```python
from build123d import *

# Parameters (mm, degrees)
SKETCH1_R           = 1.5
BOSS_EXTRUDE1_DEPTH = 5.13
SKETCH2_W           = 21.373732632
SKETCH2_H           = 5.13
BOSS_EXTRUDE2_DEPTH = 2.5
SKETCH3_W           = 21.373732632
SKETCH3_H           = 2.5
BOSS_EXTRUDE3_DEPTH = 4.6
BOSS_EXTRUDE4_START = -2.95
BOSS_EXTRUDE4_DEPTH = 2.95
CUT_EXTRUDE1_REACH  = 103.599
SKETCH5_R           = 1.75
SKETCH6_R           = 1.6
SKETCH6_R_2         = 1.5
CUT_EXTRUDE2_DEPTH  = 34.549423701
CUT_EXTRUDE3_REACH  = 103.262


with BuildPart() as part:
    # Sketch1 → Boss-Extrude1 (new body)
    with BuildSketch(Plane.XY):
        with BuildLine():
            Line((-11.282357346, 86.580844321), (-10.686866316, 72.941857381))
            Line((-10.686866316, 72.941857381), (10.686866316, 72.941857381))
            Line((10.686866316, 72.941857381), (11.282357346, 86.580844321))
            ThreePointArc((11.282357346, 86.580844321), (11.19104264, 87.774392868), (10.818655174, 88.912032567))
            Line((10.818655174, 88.912032567), (7.70361619, 95.592255225))
            ThreePointArc((7.70361619, 95.592255225), (0, 100.5), (-7.70361619, 95.592255225))
            Line((-7.70361619, 95.592255225), (-10.818655174, 88.912032567))
            ThreePointArc((-10.818655174, 88.912032567), (-11.19104264, 87.774392868), (-11.282357346, 86.580844321))
        make_face()
        with Locations((-6.25, 79)):
            Circle(SKETCH1_R, mode=Mode.SUBTRACT)
        with Locations((-6.25, 89)):
            Circle(SKETCH1_R, mode=Mode.SUBTRACT)
        with Locations((6.25, 79)):
            Circle(SKETCH1_R, mode=Mode.SUBTRACT)
        with Locations((6.25, 89)):
            Circle(SKETCH1_R, mode=Mode.SUBTRACT)
    extrude(amount=BOSS_EXTRUDE1_DEPTH)

    # Sketch2 → Boss-Extrude2 (add)
    with BuildSketch(Plane.XZ.offset(-72.941857381)):
        with Locations((0, 2.565)):
            Rectangle(SKETCH2_W, SKETCH2_H)
    extrude(amount=BOSS_EXTRUDE2_DEPTH)

    # Sketch3 → Boss-Extrude3 (add)
    with BuildSketch(Plane.XY.offset(5.13)):
        with Locations((0, 71.691857381)):
            Rectangle(SKETCH3_W, SKETCH3_H)
    extrude(amount=BOSS_EXTRUDE3_DEPTH)

    # Sketch4 → Boss-Extrude4 (add)
    with BuildSketch(Plane.XY.offset(9.73).offset(BOSS_EXTRUDE4_START)):
        with BuildLine():
            Line((4.561250463, 86.075), (2.872500925, 89))
            Line((2.872500925, 89), (4.561250463, 91.925))
            Line((4.561250463, 91.925), (-4.561250463, 91.925))
            Line((-4.561250463, 91.925), (-2.872500925, 89))
            Line((-2.872500925, 89), (-4.561250463, 86.075))
            Line((-4.561250463, 86.075), (-7.938749537, 86.075))
            Line((-7.938749537, 86.075), (-9.627499075, 89))
            Line((-9.627499075, 89), (-7.938749537, 91.925))
            Line((-7.938749537, 91.925), (-9.413685386, 91.925))
            Line((-9.413685386, 91.925), (-10.818655174, 88.912032567))
            ThreePointArc((-10.818655174, 88.912032567), (-11.19104264, 87.774392868), (-11.282357346, 86.580844321))
            Line((-11.282357346, 86.580844321), (-10.686866316, 72.941857381))
            Line((-10.686866316, 72.941857381), (10.686866316, 72.941857381))
            Line((10.686866316, 72.941857381), (11.282357346, 86.580844321))
            ThreePointArc((11.282357346, 86.580844321), (11.19104264, 87.774392868), (10.818655174, 88.912032567))
            Line((10.818655174, 88.912032567), (9.413685386, 91.925))
            Line((9.413685386, 91.925), (7.938749537, 91.925))
            Line((7.938749537, 91.925), (9.627499075, 89))
            Line((9.627499075, 89), (7.938749537, 86.075))
            Line((7.938749537, 86.075), (4.561250463, 86.075))
        make_face()
        Polygon((-4.561250463, 81.925), (-2.872500925, 79), (-4.561250463, 76.075), (-7.938749537, 76.075), (-9.627499075, 79), (-7.938749537, 81.925), align=None, mode=Mode.SUBTRACT)
        Polygon((7.938749537, 81.925), (9.627499075, 79), (7.938749537, 76.075), (4.561250463, 76.075), (2.872500925, 79), (4.561250463, 81.925), align=None, mode=Mode.SUBTRACT)
    extrude(amount=BOSS_EXTRUDE4_DEPTH)

    # Sketch5 → Cut-Extrude1 (cut, up to next)
    with BuildSketch(Plane(origin=(0, 0, 0), x_dir=(-1, 0, 0), z_dir=(0, 0, -1)), mode=Mode.PRIVATE) as cut_extrude1_sk1:
        with Locations((-6.25, 89)):
            Circle(SKETCH5_R)
    cut_extrude1_tool1 = extrude(cut_extrude1_sk1.sketch, amount=-CUT_EXTRUDE1_REACH, mode=Mode.PRIVATE) & part.part
    # Sketch5 → Cut-Extrude1 (cut, up to next)
    with BuildSketch(Plane(origin=(0, 0, 0), x_dir=(-1, 0, 0), z_dir=(0, 0, -1)), mode=Mode.PRIVATE) as cut_extrude1_sk2:
        with Locations((6.25, 89)):
            Circle(SKETCH5_R)
    cut_extrude1_tool2 = extrude(cut_extrude1_sk2.sketch, amount=-CUT_EXTRUDE1_REACH, mode=Mode.PRIVATE) & part.part
    # Sketch5 → Cut-Extrude1 (cut, up to next)
    with BuildSketch(Plane(origin=(0, 0, 0), x_dir=(-1, 0, 0), z_dir=(0, 0, -1)), mode=Mode.PRIVATE) as cut_extrude1_sk3:
        with Locations((6.25, 79)):
            Circle(SKETCH5_R)
    cut_extrude1_tool3 = extrude(cut_extrude1_sk3.sketch, amount=-CUT_EXTRUDE1_REACH, mode=Mode.PRIVATE) & part.part
    # Sketch5 → Cut-Extrude1 (cut, up to next)
    with BuildSketch(Plane(origin=(0, 0, 0), x_dir=(-1, 0, 0), z_dir=(0, 0, -1)), mode=Mode.PRIVATE) as cut_extrude1_sk4:
        with Locations((-6.25, 79)):
            Circle(SKETCH5_R)
    cut_extrude1_tool4 = extrude(cut_extrude1_sk4.sketch, amount=-CUT_EXTRUDE1_REACH, mode=Mode.PRIVATE) & part.part
    add(cut_extrude1_tool1.solids().sort_by_distance((6.25, 89, 0))[0], mode=Mode.SUBTRACT)
    add(cut_extrude1_tool2.solids().sort_by_distance((-6.25, 89, 0))[0], mode=Mode.SUBTRACT)
    add(cut_extrude1_tool3.solids().sort_by_distance((-6.25, 79, 0))[0], mode=Mode.SUBTRACT)
    add(cut_extrude1_tool4.solids().sort_by_distance((6.25, 79, 0))[0], mode=Mode.SUBTRACT)

    # Sketch6 → Cut-Extrude2 (cut, through all)
    with BuildSketch(Plane.XZ.offset(-70.441857381)):
        with Locations(Location((0, 2.565, 0), (0, 0, 270))):
            Circle(SKETCH6_R)
        with Locations((-10, 2.565)):
            Circle(SKETCH6_R_2)
        with Locations((10, 2.565)):
            Circle(SKETCH6_R_2)
    extrude(amount=-CUT_EXTRUDE2_DEPTH, mode=Mode.SUBTRACT)

    # Sketch7 → Cut-Extrude3 (cut, up to next)
    with BuildSketch(Plane.XY.offset(5.13), mode=Mode.PRIVATE) as cut_extrude3_sk1:
        with BuildLine():
            Line((-7.70361619, 95.592255225), (-9.413685386, 91.925))
            Line((-9.413685386, 91.925), (9.413685386, 91.925))
            Line((9.413685386, 91.925), (7.70361619, 95.592255225))
            ThreePointArc((7.70361619, 95.592255225), (0, 100.5), (-7.70361619, 95.592255225))
        make_face()
    cut_extrude3_tool1 = extrude(cut_extrude3_sk1.sketch, amount=-CUT_EXTRUDE3_REACH, mode=Mode.PRIVATE) & part.part
    add(cut_extrude3_tool1.solids().sort_by_distance((0, 95.513825, 5.13))[0], mode=Mode.SUBTRACT)


solid = part.part
```
Can you work these out from the model? Positions are in its coordinate system, mm. A direction names the side the tool comes from. Give positions to 0.01 mm unless a question says otherwise; leave off trailing zeros. Write each loop counter-clockwise with the first axis right and the second up, starting at its lowest first coordinate (ties: lowest second). Pieces come first, ordered by that corner, then holes. Notation, with made-up numbers: (34, -17.5) - (75, -17.5) arc R11 cw to (75, 2.5) - close; hole circle Ø11 at (-36, 61.5). An arc over 180 degrees is marked (long way). Write item = value, one per line. Start each with the question number.
1. For pin 1 (0.6 mm diameter, centred on y = 71.5, z = 0.5, fed in from -X); pin 2 (1.5 mm diameter, centred on y = 83.5, z = 8, fed in from +X); pin 3 (1.4 mm diameter, centred on y = 72, z = 0.5, fed in from +X), each with a flat end and sliding along its axis, tell me the tip position at first contact or that it passes through.
2. On a 3-axis mill with a long thin cutter (end or side, diameter ignored), from which of +Z, -Z, +X, -X, +Y, -Y can I reach the whole of each face in a straight line? I mean faces 5 (the face through (-10.99, 79.86, 4.42)), 6 (the face through (-6, 81.925, 8)). Say none if no direction works.
3. Imagine slicing it at B-B (z = 2.75). Please give me the cut outline in (x, y) (3 decimals).
4. Thinking about a two-plate mould opening in Z: for faces 1 (the face through (-8.5, 81, 2.5)), 2 (the face through (0, 81, 0)), 3 (the face through (-1.562, 81.033, 2.912)), 4 (the face through (3.729, 77.517, 8.234)), which applies, released by +Z, released by -Z, zero draft, split by the parting line, or undercut?
5. Imagine slicing it at C-C (y = 85). Please give me the cut outline in (x, z) (3 decimals), and give its area (3 significant figures).
6. Please list where these lines run through material, in increasing order: line 1 (Z direction, x = 3.25, y = 74.5); line 2 (Y direction, x = 6.25, z = 2.6) (3 decimals); line 3 (Y direction, x = 6, z = 8.25) (3 decimals).
7. Imagine slicing it at D-D (x = 0). Please give me the cut outline in (y, z) (3 decimals), and give its area (3 significant figures).
8. Imagine slicing it at A-A (x = -6.25). Please give me the cut outline in (y, z) (3 decimals), and give its area (3 significant figures).
Worked answers:
q1.pin_1 = -10.69
q1.pin_2 = 11.18
q1.pin_3 = 10.69
q2.face_5 = +Z, -Z, -X, -Y
q2.face_6 = +Z
q3.outline = (-8.511, 70.442) - (-1.589, 70.442) - (-1.589, 91.925) - (-8.511, 91.925) - close; (1.589, 70.442) - (8.511, 70.442) - (8.511, 91.925) - (1.589, 91.925) - close; hole circle Ø3.5 at (-6.25, 79); hole circle Ø3.5 at (-6.25, 89); hole circle Ø3.5 at (6.25, 79); hole circle Ø3.5 at (6.25, 89)
q4.face_1 = undercut
q4.face_2 = released by -Z
q4.face_3 = undercut
q4.face_4 = zero draft
q5.outline = (-11.213, 0) - (11.213, 0) - (11.213, 1.683) arc R1.5 cw (long way) to (11.213, 3.447) - (11.213, 5.13) - (-11.213, 5.13) - (-11.213, 3.447) arc R1.5 cw (long way) to (-11.213, 1.683) - close; (-11.213, 6.78) - (11.213, 6.78) - (11.213, 9.73) - (-11.213, 9.73) - close; hole circle Ø3.2 at (0, 2.565)
q5.area = 160 mm2
q6.line_1 = 0 to 5.13, 6.78 to 9.73
q6.line_2 = 70.442 to 77.25, 80.75 to 87.25, 90.75 to 91.925
q6.line_3 = 70.442 to 76.075, 81.925 to 86.075
q7.outline = (70.442, 0) - (91.925, 0) - (91.925, 0.965) - (70.442, 0.965) - close; (70.442, 4.165) - (91.925, 4.165) - (91.925, 5.13) - (72.942, 5.13) - (72.942, 6.78) - (91.925, 6.78) - (91.925, 9.73) - (70.442, 9.73) - close
q7.area = 109 mm2
q8.outline = (70.442, 0) - (77.25, 0) - (77.25, 5.13) - (72.942, 5.13) - (72.942, 6.78) - (76.075, 6.78) - (76.075, 9.73) - (70.442, 9.73) - close; (80.75, 0) - (87.25, 0) - (87.25, 5.13) - (80.75, 5.13) - close; (81.925, 6.78) - (86.075, 6.78) - (86.075, 9.73) - (81.925, 9.73) - close; (90.75, 0) - (91.925, 0) - (91.925, 5.13) - (90.75, 5.13) - close
q8.area = 107 mm2
